Part model, mm, in its own coordinate system. Face numbers are marked on the shaded views. A direction names the side the tool comes from. Give positions to 0.01 mm unless a question says otherwise; leave off trailing zeros. Write each loop counter-clockwise with the first axis right and the second up, starting at its lowest first coordinate (ties: lowest second). Pieces come first, ordered by that corner, then holes.
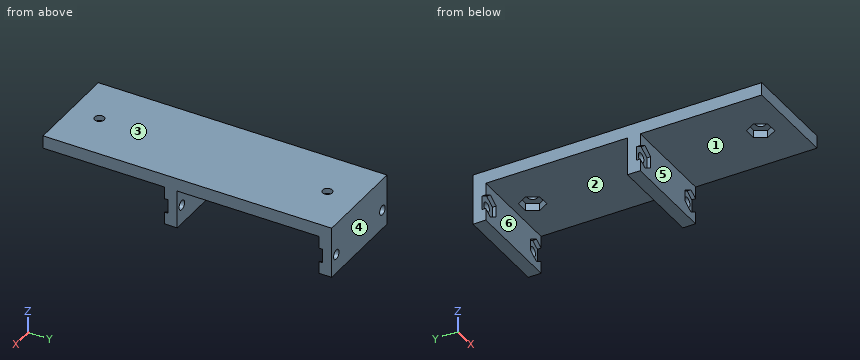
```python
from build123d import *

# Parameters (mm, degrees)
EXTRU_MINCE1_START      = -19.05
EXTRU_MINCE1_DEPTH      = 38.1
ESQUISSE3_R             = 1.89865
ENL_V_MAT_EXTRU_2_DEPTH = 75.865138463
D_GAGEMENT_61_D         = 3.7973
ENL_V_MAT_EXTRU_3_DEPTH = 3
ENL_V_MAT_EXTRU_4_DEPTH = 1.5
ENL_V_MAT_EXTRU_5_DEPTH = 1.5


# Read off the part's stored shape, not the designer's step: Extru.-Mince1
with BuildPart() as part:
    # Extru.-Mince1 outline → Extru.-Mince1 (new body)
    with BuildSketch(Plane(origin=(0, 0, 0), x_dir=(0, 0, -1), z_dir=(1, 0, 0)).offset(EXTRU_MINCE1_START)):
        Polygon((20.32, -16.1508919), (5.08, -16.1508919), (5.08, 40.1736081), (20.32, 40.1736081), (20.32, 45.2536081), (0, 45.2536081), (0, -69.4908919), (5.08, -69.4908919), (5.08, -21.2308919), (20.32, -21.2308919), align=None)
    extrude(amount=EXTRU_MINCE1_DEPTH)

    # Esquisse3 → Enlèv. mat.-Extru.2 (cut, through all)
    with BuildSketch(Plane.XY):
        with Locations((0, -58.0608919)):
            Circle(ESQUISSE3_R)
        with Locations((0, 32.5536081)):
            Circle(ESQUISSE3_R)
    extrude(amount=-ENL_V_MAT_EXTRU_2_DEPTH, mode=Mode.SUBTRACT)

    # Dégagement #61 (through all)
    with Locations(Plane(origin=(0, -21.2308919, 0), x_dir=(-1, 0, 0), z_dir=(0, -1, 0))):
        with Locations((-15.875, 12.7), (15.875, 12.7)):
            Hole(D_GAGEMENT_61_D / 2)

    # Esquisse10 → Enlèv. mat.-Extru.3 (cut)
    with BuildSketch(Plane(origin=(0, 0, -5.08), x_dir=(-1, 0, 0), z_dir=(0, 0, -1))):
        Polygon((2.453738644, 36.8036081), (-2.453738644, 36.8036081), (-4.907477288, 32.5536081), (-2.453738644, 28.3036081), (2.453738644, 28.3036081), (4.907477288, 32.5536081), align=None)
        Polygon((2.453738644, -53.8108919), (-2.453738644, -53.8108919), (-4.907477288, -58.0608919), (-2.453738644, -62.3108919), (2.453738644, -62.3108919), (4.907477288, -58.0608919), align=None)
    extrude(amount=-ENL_V_MAT_EXTRU_3_DEPTH, mode=Mode.SUBTRACT)

    # Esquisse12 → Enlèv. mat.-Extru.4 (cut)
    with BuildSketch(Plane.XZ.offset(21.2308919)):
        Polygon((11.875, -10.390598923), (11.875, -15.009401077), (15.875, -17.318802154), (19.875, -15.009401077), (19.875, -10.390598923), (15.875, -8.081197846), align=None)
        Polygon((-19.875, -10.390598923), (-19.875, -15.009401077), (-15.875, -17.318802154), (-11.875, -15.009401077), (-11.875, -10.390598923), (-15.875, -8.081197846), align=None)
    extrude(amount=-ENL_V_MAT_EXTRU_4_DEPTH, mode=Mode.SUBTRACT)

    # Esquisse13 → Enlèv. mat.-Extru.5 (cut)
    with BuildSketch(Plane.XZ.offset(-40.1736081)):
        Polygon((-11.875, -15.009401077), (-11.875, -10.390598923), (-15.875, -8.081197846), (-19.875, -10.390598923), (-19.875, -15.009401077), (-15.875, -17.318802154), align=None)
        Polygon((15.875, -8.081197846), (11.875, -10.390598923), (11.875, -15.009401077), (15.875, -17.318802154), (19.875, -15.009401077), (19.875, -10.390598923), align=None)
    extrude(amount=-ENL_V_MAT_EXTRU_5_DEPTH, mode=Mode.SUBTRACT)


solid = part.part
```
1) Saw through at C-C, the plane z = -3.75. Write the cut outline in (x, y), then the cut area to 3 significant figures.
Answers follow:
outline: (-19.05, -69.49) - (19.05, -69.49) - (19.05, 45.25) - (-19.05, 45.25) - close; hole (-4.91, -58.06) - (-2.45, -62.31) - (2.45, -62.31) - (4.91, -58.06) - (2.45, -53.81) - (-2.45, -53.81) - close; hole (-4.91, 32.55) - (-2.45, 28.3) - (2.45, 28.3) - (4.91, 32.55) - (2.45, 36.8) - (-2.45, 36.8) - close
area: 4,250 mm2
2) 3-axis set-ups, long thin cutter, end or side, ignore diameter. For the marked faces 1, 2 and 3: which of +Z, -Z, +X, -X, +Y, -Y reach the whole face in a straight line?
Answers follow:
face 1: -Z, +X, -X, -Y
face 2: -Z, +X, -X
face 3: +Z, +X, -X, +Y, -Y
3) Two-plate mould, pull along Y, no slides. Class the marked faces 4, 5 and 6: +Y half, -Y half, draft (parallel to the pull), parting line (faces both ways), or undercut.
Answers follow:
face 4: +Y half
face 5: -Y half
face 6: undercut
4) Saw through at D-D, the plane y = 16. Write the cut outline in (x, z).
Answers follow:
outline: (-19.05, -5.08) - (19.05, -5.08) - (19.05, 0) - (-19.05, 0) - close
5) Pin check, flat tips, straight feed: pin 1 Ø0.8 at (y, z) = (-20.5, -11.5) entering from +X (3 decimals); pin 2 Ø5 at (x, z) = (15.875, -12.7) entering from -Y; pin 3 Ø5.5 at (x, z) = (14, -13.5) entering from -Y; pin 4 Ø2.5 at (x, y) = (0, -58.06) entering from -Z. Stop position of each tip, or through.
Answers follow:
pin 1: stops at x = 11.875
pin 2: stops at y = -19.73
pin 3: stops at y = -21.23
pin 4: passes through
6) Saw through at B-B, the plane z = -12.7. Count the separate pieces of the cut face and the enclosed holes in it, then the cut area to 3 significant figures.
Answers follow:
separate pieces: 6
enclosed holes: 0
area: 290 mm2
7) Saw through at A-A, the plane x = 0. Write the cut outline in (y, z).
Answers follow:
outline: (-69.49, -5.08) - (-62.31, -5.08) - (-62.31, -2.08) - (-59.96, -2.08) - (-59.96, 0) - (-69.49, 0) - close; (-56.16, -2.08) - (-53.81, -2.08) - (-53.81, -5.08) - (-21.23, -5.08) - (-21.23, -20.32) - (-16.15, -20.32) - (-16.15, -5.08) - (28.3, -5.08) - (28.3, -2.08) - (30.65, -2.08) - (30.65, 0) - (-56.16, 0) - close; (34.45, -2.08) - (36.8, -2.08) - (36.8, -5.08) - (40.17, -5.08) - (40.17, -20.32) - (45.25, -20.32) - (45.25, 0) - (34.45, 0) - close
8) Wall check: L1, parallel to X at y = 43.6, z = -12.7; L2, parallel to Y at x = 0, z = -0.55; L3, parallel to Y at x = 7, z = -7.75. Give the ranges that are in metal, low to high.
Answers follow:
L1: x = -19.05 to -17.77, -13.98 to 13.98, 17.77 to 19.05
L2: y = -69.49 to -59.96, -56.16 to 30.65, 34.45 to 45.25
L3: y = -21.23 to -16.15, 40.17 to 45.25
